from build123d import *

# Parameters (mm, degrees)
EXTRUDE_1_DEPTH          = 14
EXTRUDE_START            = 10
EXTRUDE_2_DEPTH          = 10
CUT_EXTRUDE_1_DEPTH      = 104.831594421
CUT_EXTRUDE_1_DEPTH_BACK = 104.831594421
SKETCH_3_R               = 2
SKETCH_4_R               = 2.65
CUT_EXTRUDE_2_DEPTH      = 104.831594421
SKETCH_6_W               = 2
SKETCH_6_H               = 24
CUT_EXTRUDE_3_DEPTH      = 2
SKETCH_7_W               = 2
SKETCH_7_H               = 24
CUT_EXTRUDE_4_DEPTH      = 2
SKETCH_8_W               = 2
SKETCH_8_H               = 28
CUT_EXTRUDE_5_DEPTH      = 2
CUT_EXTRUDE_6_DEPTH      = 104.831594421
CUT_EXTRUDE_6_DEPTH_BACK = 104.831594421
SKETCH_9_W               = 2
SKETCH_9_H               = 1
SKETCH_10_W              = 9.2
SKETCH_10_H              = 6.7
CUT_EXTRUDE_7_DEPTH      = 4


with BuildPart() as part:
    # Sketch 2 → Extrude 1 (new body)
    with BuildSketch(Plane.XY):
        with BuildLine():
            Line((-85, 14), (0, 14))
            ThreePointArc((0, 14), (14, 0), (0, -14))
            Line((0, -14), (-85, -14))
            ThreePointArc((-85, -14), (-99, 0), (-85, 14))
        make_face()
        with BuildLine():
            Line((-26.5, -8), (-58.5, -8))
            ThreePointArc((-58.5, -8), (-66.5, 0), (-58.5, 8))
            Line((-58.5, 8), (-26.5, 8))
            ThreePointArc((-26.5, 8), (-18.5, 0), (-26.5, -8))
        make_face(mode=Mode.SUBTRACT)
        Polygon((-84.5, 3.05), (-84.5, -3.45), (-75.481671923, -3.45), (-75.3, -3.45), (-75.3, 3.25), (-75.481671923, 3.25), (-84.5, 3.25), align=None, mode=Mode.SUBTRACT)
        Polygon((-9.7, 3.25), (-9.518328077, 3.25), (-0.5, 3.25), (-0.5, 3.05), (-0.5, -3.45), (-9.518328077, -3.45), (-9.7, -3.45), align=None, mode=Mode.SUBTRACT)
    extrude(amount=-EXTRUDE_1_DEPTH)

    # Sketch 2_3 → Extrude 2 (add)
    with BuildSketch(Plane.XY.offset(EXTRUDE_START)):
        with BuildLine():
            Line((0, 14), (-85, 14))
            ThreePointArc((-85, 14), (-99, 0), (-85, -14))
            Line((-85, -14), (0, -14))
            ThreePointArc((0, -14), (14, 0), (0, 14))
        make_face()
        with BuildLine():
            ThreePointArc((-26.5, 8), (-18.5, 0), (-26.5, -8))
            Line((-26.5, -8), (-58.5, -8))
            ThreePointArc((-58.5, -8), (-66.5, 0), (-58.5, 8))
            Line((-58.5, 8), (-26.5, 8))
        make_face(mode=Mode.SUBTRACT)
    extrude(amount=-EXTRUDE_2_DEPTH)

    # Sketch 3 → Cut-Extrude 1 (cut, two sides: drawn at the far end of the back side and taken through both)
    with BuildSketch(Plane(origin=(0, 14, 0), x_dir=(1, 0, 0), z_dir=(0, 1, 0)).offset(-CUT_EXTRUDE_1_DEPTH_BACK)):
        with Locations(Location((-5, 5, 0), (0, 0, 270))):
            Circle(SKETCH_3_R)
        with Locations(Location((-80, 5, 0), (0, 0, 270))):
            Circle(SKETCH_3_R)
    extrude(amount=CUT_EXTRUDE_1_DEPTH + CUT_EXTRUDE_1_DEPTH_BACK, mode=Mode.SUBTRACT)

    # Sketch 4 → Cut-Extrude 2 (cut, through all)
    with BuildSketch(Plane(origin=(0, 14, 0), x_dir=(1, 0, 0), z_dir=(0, 1, 0))):
        with Locations(Location((-42.5, -0.15, 0), (0, 0, 270))):
            Circle(SKETCH_4_R)
    extrude(amount=-CUT_EXTRUDE_2_DEPTH, mode=Mode.SUBTRACT)

    # Sketch 6 → Cut-Extrude 3 (cut)
    with BuildSketch(Plane(origin=(0, 14, 0), x_dir=(1, 0, 0), z_dir=(0, 1, 0))):
        with Locations((-11, 2)):
            Rectangle(SKETCH_6_W, SKETCH_6_H)
    cut_extrude_3 = extrude(amount=-CUT_EXTRUDE_3_DEPTH, mode=Mode.SUBTRACT)

    # Mirror 1: Cut-Extrude 3 across plane
    add(cut_extrude_3.mirror(Plane.ZX), mode=Mode.SUBTRACT)

    # Sketch 7 → Cut-Extrude 4 (cut)
    with BuildSketch(Plane(origin=(0, 14, 0), x_dir=(1, 0, 0), z_dir=(0, 1, 0))):
        with Locations((-74, 2)):
            Rectangle(SKETCH_7_W, SKETCH_7_H)
    cut_extrude_4 = extrude(amount=-CUT_EXTRUDE_4_DEPTH, mode=Mode.SUBTRACT)

    # Mirror 2: Cut-Extrude 4 across plane
    add(cut_extrude_4.mirror(Plane.ZX), mode=Mode.SUBTRACT)

    # Sketch 8 → Cut-Extrude 5 (cut)
    with BuildSketch(Plane.XY.offset(10)):
        with Locations((-11, 0)):
            Rectangle(SKETCH_8_W, SKETCH_8_H)
        with Locations((-74, 0)):
            Rectangle(SKETCH_8_W, SKETCH_8_H)
    extrude(amount=-CUT_EXTRUDE_5_DEPTH, mode=Mode.SUBTRACT)

    # Sketch 9 → Cut-Extrude 6 (cut, two sides: drawn at the far end of the back side and taken through both)
    with BuildSketch(Plane.XZ.offset(14).offset(-CUT_EXTRUDE_6_DEPTH_BACK)):
        with Locations((-74, -13.5)):
            Rectangle(SKETCH_9_W, SKETCH_9_H)
        with Locations((-11, -13.5)):
            Rectangle(SKETCH_9_W, SKETCH_9_H)
    extrude(amount=CUT_EXTRUDE_6_DEPTH + CUT_EXTRUDE_6_DEPTH_BACK, mode=Mode.SUBTRACT)

    # Sketch 10 → Cut-Extrude 7 (cut)
    with BuildSketch(Plane(origin=(0, 0, 0), x_dir=(-1, 0, 0), z_dir=(0, 0, -1))):
        with Locations((79.9, -0.1)):
            Rectangle(SKETCH_10_W, SKETCH_10_H)
        with Locations((5.1, -0.1)):
            Rectangle(SKETCH_10_W, SKETCH_10_H)
    extrude(amount=-CUT_EXTRUDE_7_DEPTH, mode=Mode.SUBTRACT)


solid = part.part
Verification items for the finished model (mm, model axes). A direction names the side the tool comes from. Give positions to 0.01 mm unless a question says otherwise; leave off trailing zeros. Order: outer loops, then holes, each group sorted by start corner. A loop starts at its lowest first (then second) coordinate and runs counter-clockwise, first axis right, second up. Notation, with made-up numbers: M 67,-33 L 79,-33 A6 cw 79,-27 Z; hole C 54.25,37 d3. An arc over 180 degrees is marked long. Use one line per item in the form item = value. Start each with the question number.
Q1. Section check C-C (y = 4.75). Enter the section's corners in (x, z), then the cut area to 3 significant figures.
Q2. Scan lines: line 1 along Z through (x, y) = (-80, -8.5); line 2 along X through (y, z) = (9.5, -5); line 3 along X through (y, z) = (-3.25, -10.25). Record each from-to range of solid material in increasing order. Write a range as [from, to].
Q3. Section check D-D (x = -42.5). Enter the section's corners in (y, z).
Q4. Go/stop test with flat-tipped pins: pin 1 Ø2 at (y, z) = (8.5, -10.5) entering from +X; pin 2 Ø1 at (x, y) = (-74, 2) entering from -Z; pin 3 Ø3 at (x, z) = (-80, -5) entering from -Y; pin 4 Ø1 at (x, y) = (-11, -4.5) entering from +Z. Record where each tip stops, or that it passes through.
Q5. Section check B-B (x = -5). Enter the section's corners in (y, z), then the cut area to 3 significant figures.
Q6. Mould release check, pull along Z, two halves, no side actions. Record for faces 1 (the flat face through (-87, 0, -14)), 2 (the flat face through (-43, 8, -4)), 3 (the cylindrical face through (-78, 9, -5)): +Z half, -Z half, draft (parallel to the pull), parting line (faces both ways), or undercut.
Q7. Access from +Z, -Z, +X, -X, +Y, -Y to the whole of each face (thin tool, end or side, straight path). Record for faces 4 (the flat face through (-42, -8, -4)), 5 (the flat face through (-12, 1, 9)), 6 (the flat face through (-11, -12, -3)), 7 (the flat face through (-74, 12, -3)), 8 (the flat face through (-84.5, 0, -5)).
Evaluation:
q1.outline = M -98.17,-14 L -75,-14 L -75,-13 L -73,-13 L -73,-14 L -64.94,-14 L -64.94,10 L -73,10 L -73,8 L -75,8 L -75,10 L -98.17,10 Z; M -20.06,-14 L -12,-14 L -12,-13 L -10,-13 L -10,-14 L 13.17,-14 L 13.17,10 L -10,10 L -10,8 L -12,8 L -12,10 L -20.06,10 Z; hole C -80,-5 d4; hole C -5,-5 d4
q1.area = 1,560 mm2
q2.line_1 = [-14, -7], [-3, 10]
q2.line_2 = [-95.28, -82], [-78, -7], [-3, 10.28]
q2.line_3 = [-98.62, -84.5], [-75.3, -65.81], [-19.19, -9.7], [-0.5, 13.62]
q3.outline = M -14,-14 L -8,-14 L -8,-2.5 L -14,-2.5 Z; M -14,2.8 L -8,2.8 L -8,10 L -14,10 Z; M 8,-14 L 14,-14 L 14,-2.5 L 8,-2.5 Z; M 8,2.8 L 14,2.8 L 14,10 L 8,10 Z
q4.pin_1 = 11.82
q4.pin_2 = -13
q4.pin_3 = through
q4.pin_4 = 8
q5.outline = M -14,-14 L -3.45,-14 L -3.45,-7 L -14,-7 Z; M -14,-3 L -3.45,-3 L -3.45,4 L 3.25,4 L 3.25,-3 L 14,-3 L 14,10 L -14,10 Z; M 3.25,-14 L 14,-14 L 14,-7 L 3.25,-7 Z
q5.area = 466 mm2
q6.face_1 = -Z half
q6.face_2 = draft
q6.face_3 = undercut
q7.face_4 = +Z, -Z
q7.face_5 = none
q7.face_6 = +Z, -Z, -Y
q7.face_7 = +Z, -Z, +Y
q7.face_8 = -Z
